Can you work these out from the drawing? Everything is in mm from the part's minimum corner. Round coordinates to 2 decimals unless told otherwise and drop trailing zeros. Loops run counter-clockwise (first coordinate to the right, second up) from the corner with the lowest first, then second, coordinate; pieces in that order, holes last. Notation, with made-up numbers: (1.25, 85) - (34.25, 85) arc R24 cw to (34.25, 114) - close; hole circle Ø11 at (4, 2.25). An arc over 180 degrees is marked (long way). Answer as CSV lines item,"result". Start each with the question number.
1) Please list where these lines run through material, in increasing order: line 1 along Z through (x, y) = (25.6, 36.75); line 2 along Z through (x, y) = (45, 9.5); line 3 along Y through (x, z) = (39, 29) (1 decimal).
2) I'm going to push flat-ended pins straight in: pin 1 Ø1.5 at (x, z) = (10, 4.5) entering from -Y (1 decimal); pin 2 Ø12 at (x, z) = (8.5, 31) entering from -Y; pin 3 Ø3 at (x, y) = (19.5, 30) entering from +Z. Where does each tip first touch, or does it pass through?
3) Suppose I cut it at C-C, the plane x = 46.5. Write out the boundary of the cut face in (y, z).
4) Suppose I cut it at B-B, the plane x = 25.6. Write out the boundary of the cut face in (y, z), then the cut area to 3 significant figures.
5) We'd pull the mould along Z, two halves only. Please class the marked faces 1, 2 and 3: pulls with the +Z half, pulls with the -Z half, needs draft (parallel to the pull), parting line crosses it, or undercut.
6) Suppose I cut it at D-D, the plane z = 13. Count the separate pieces of the cut face and the enclosed holes in it, then the cut area to 3 significant figures.
7) Suppose I cut it at A-A, the plane z = 17.9. Write out the boundary of the cut face in (x, y).
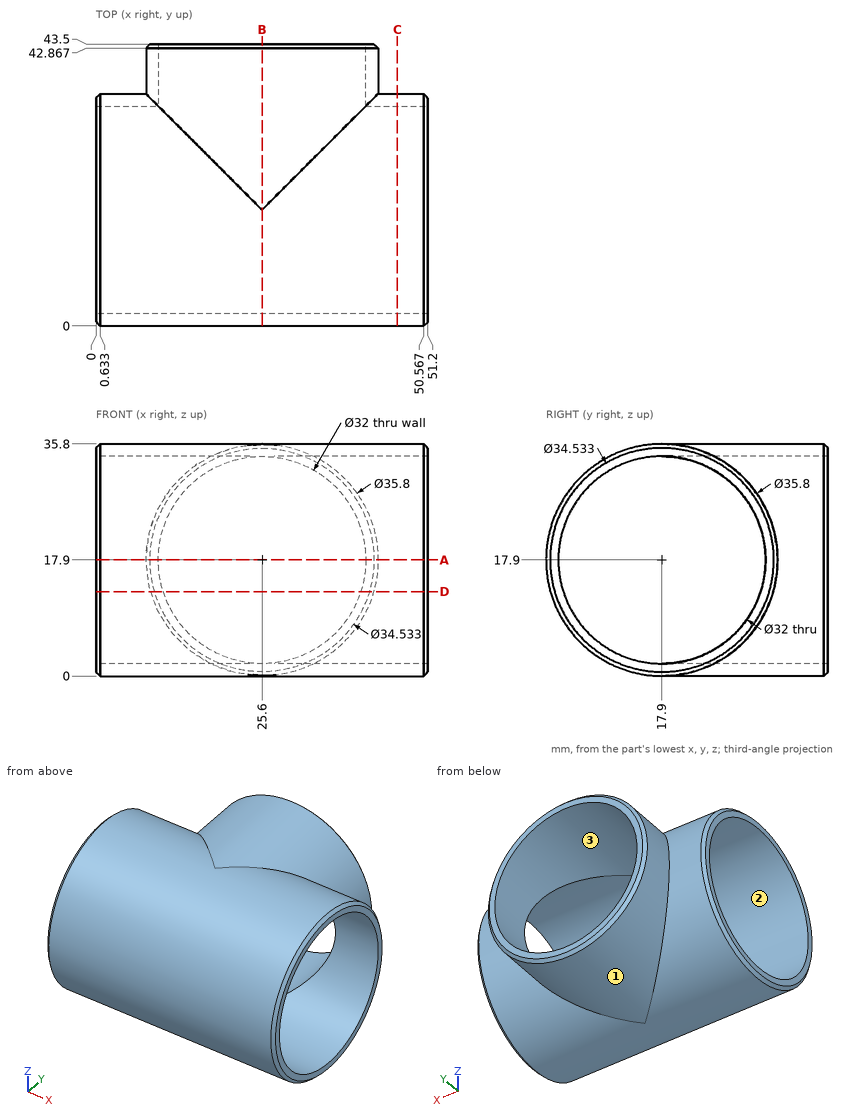
Filled sheet:
1,line 1,"0 to 1.9, 33.9 to 35.8"
1,line 2,"2.09 to 4.28, 31.52 to 33.71"
1,line 3,"3.9 to 6.4, 29.4 to 43.4"
2,pin 1,"y = 5.2"
2,pin 2,"y = 1.47"
2,pin 3,"z = 35.2"
3,outline,"circle Ø35.8 at (17.9, 17.9); hole circle Ø32 at (17.9, 17.9)"
4,outline,"(17.9, 0) - (42.87, 0) - (43.5, 0.63) - (43.5, 1.9) - (17.9, 1.9) arc R16 cw to (17.9, 33.9) - (43.5, 33.9) - (43.5, 35.17) - (42.87, 35.8) - (17.9, 35.8) arc R17.9 ccw to start"
4,area,"198 mm²"
5,face 1,"parting line crosses it"
5,face 2,"undercut"
5,face 3,"undercut"
6,separate pieces,"3"
6,enclosed holes,"0"
6,area,"175 mm²"
7,outline,"(0, 0.63) - (0.63, 0) - (50.57, 0) - (51.2, 0.63) - (51.2, 1.9) - (0, 1.9) - close; (0, 33.9) - (9.6, 33.9) - (9.6, 43.5) - (8.33, 43.5) - (7.7, 42.87) - (7.7, 35.8) - (0.63, 35.8) - (0, 35.17) - close; (41.6, 33.9) - (51.2, 33.9) - (51.2, 35.17) - (50.57, 35.8) - (43.5, 35.8) - (43.5, 42.87) - (42.87, 43.5) - (41.6, 43.5) - close"
